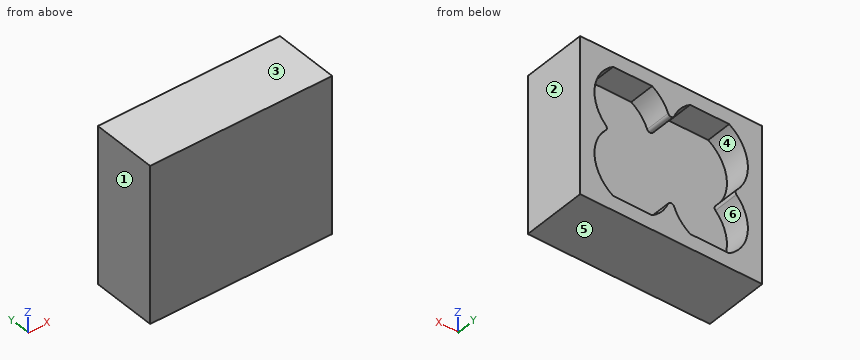
Autodesk Inventor part; units mm, degrees
ref_plane "YZ Plane" through (0, 0, 0) normal (1, 0, 0) x (0, 1, 0)
ref_plane "XZ Plane" through (0, 0, 0) normal (0, 1, 0) x (-1, 0, 0)
ref_plane "XY Plane" through (0, 0, 0) normal (0, 0, 1) x (1, 0, 0)
sketch "Sketch1" plane through (0, 0, 0) normal (0, 1, 0) x (-1, 0, 0)
  line L0 (7, 6) -> (-7, 6)
  line L1 (-7, 6) -> (-7, -6)
  line L2 (-7, -6) -> (7, -6)
  line L3 (7, -6) -> (7, 6)
  line L4 (7, 6) -> (-7, -6) construction
  line L5 (-7, 6) -> (7, -6) construction
  line L6 (4.3106, 4.4) -> (1.6094, 4.4) construction
  line L7 (1.6094, 4.4) -> (1.6094, 0.23) construction
  line L8 (1.6094, 0.23) -> (4.3106, 0.23) construction
  line L9 (4.3106, 0.23) -> (4.3106, 4.4) construction
  line L10 (4.3106, 4.4) -> (1.6094, 0.23) construction
  line L11 (1.6094, 4.4) -> (4.3106, 0.23) construction
  arc A0 (4.3106, 0.23) -> (4.3106, 4.4) centre (2.86, 2.315) ccw construction
  arc A1 (1.6094, 4.4) -> (1.6094, 0.23) centre (3.06, 2.315) ccw construction
  point P0 (0, 0)
  point P1 (2.96, 2.315)
  dimension "d0" = 12
  dimension "d1" = 14
  dimension "d2" = 4.17
  dimension "d3" = 2.54
  dimension "d4" = 4.88
  dimension "d6" = 1.6
  dimension "d7" = 1.6
extrude "Extrusion1" add sketch "Sketch1" against normal blind 5
sketch "Sketch2" plane through (0, 0, 0) normal (0, 1, 0) x (1, 0, 0)
  line L0 (-4.3106, -4.4) -> (-1.6094, -4.4) construction
  arc A0 (-4.3106, -0.23) -> (-4.3106, -4.4) centre (-2.86, -2.315) ccw construction
  arc A1 (-1.6094, -4.4) -> (-1.6094, -0.23) centre (-3.06, -2.315) ccw construction
  arc A2 (-4.8304, 0) -> (-4.4598, -4.9) centre (-2.86, -2.315) ccw
  line L1 (-4.4598, -4.9) -> (-1.4602, -4.9)
  arc A3 (-1.4602, -4.9) -> (-0.02, -2.315) centre (-3.06, -2.315) ccw
  line L2 (-7, 6) -> (-7, -6)
  line L3 (-7, -6) -> (7, -6)
  line L4 (-4.8304, 0) -> (-6.4599, 0)
  line L5 (-6.4599, 0) -> (-6.4599, -5.558) construction
  line L6 (-6.4599, -5.558) -> (0, -5.558) construction
  line L7 (0, -5.558) -> (0, -2.315) construction
  line L8 (0, -2.315) -> (-0.02, -2.315)
  line L9 (0, 8.4) -> (0, -8.4)
  line L10 (0, -2.315) -> (0, 0)
  line L11 (-4.8304, 0) -> (0, 0)
  dimension "d10" = 0.5
extrude "Extrusion2" cut sketch "Sketch2" against normal blind 2
mirror "Mirror1" about plane through (0, 0, 0) normal (0, 0, 1) of "Extrusion2"
mirror "Mirror2" about plane through (0, 0, 0) normal (1, 0, 0) of "Extrusion2", "Mirror1"
fillet "Fillet1" radius 0.25 6 edges at (-4.8304, -1, 0) (0.02, -1, 2.315) (0.02, -1, -2.315) (-0.02, -1, 2.315) (-0.02, -1, -2.315) (4.8304, -1, 0)
properties part number "ldr_case"
Geometry check sheet. Reference: the model listing, model coordinates, mm. Face numbers are marked on the shaded views. A direction names the side the tool comes from. Give positions to 0.01 mm unless a question says otherwise; leave off trailing zeros. Write each loop counter-clockwise with the first axis right and the second up, starting at its lowest first coordinate (ties: lowest second). Pieces come first, ordered by that corner, then holes. Notation, with made-up numbers: M 42.25,41 L 73.25,41 A22 cw 73.25,70 Z; hole C 31.25,88.25 d6. An arc over 180 degrees is marked long. Answer as CSV lines item,"result". Start each with the question number.
Q1. Section check B-B, the plane x = 1. Record the cut outline in (y, z), then the cut area to 3 significant figures.
Q2. Section check C-C, the plane z = -2.25. Record the cut outline in (x, y), then the cut area to 3 significant figures.
Q3. Go/stop test with a flat-tipped pin: pin 1 (3 mm diameter, centred on x = 2, z = -0.5, fed in from +Y). Record where the tip stops, or that it passes through.
Q4. Material ranges on L1, parallel to Z at x = 4, y = -1.35; L2, parallel to Z at x = -5.25, y = -0.85; L3, parallel to Y at x = 2.75, z = 4.75, recorded low to high.
Q5. Release check for a two-part mould opening along X. For the marked faces 1, 2, 3 and 4 record: pulls with the +X half, pulls with the -X half, needs draft (parallel to the pull), parting line crosses it, or undercut.
Q6. Tool access check on the marked faces 5 and 6. Record the directions out of +Z, -Z, +X, -X, +Y, -Y that give a thin tool (end or side, any length) a straight path to the whole face; none if there is none.
Geometry says:
1,outline,"M -5,-6 L 0,-6 L 0,-4.55 L -2,-4.55 L -2,4.55 L 0,4.55 L 0,6 L -5,6 Z"
1,area,"41.8 mm^2"
2,outline,"M -7,-5 L 7,-5 L 7,0 L 5.9,0 L 5.9,-2 L -5.9,-2 L -5.9,0 L -7,0 Z"
2,area,"46.4 mm^2"
3,pin 1,"y = -2"
4,L1,"-6 to -4.9, 4.9 to 6"
4,L2,"-6 to -4.19, -0.44 to 0.44, 4.19 to 6"
4,L3,"-5 to -2"
5,face 1,"pulls with the -X half"
5,face 2,"pulls with the +X half"
5,face 3,"needs draft"
5,face 4,"undercut"
6,face 5,"-Z, +X, -X, +Y, -Y"
6,face 6,"+Y"
